Can you work these out from the model? Positions are in its coordinate system, mm. Round coordinates to 2 decimals unless told otherwise and drop trailing zeros. Loops run counter-clockwise (first coordinate to the right, second up) from the corner with the lowest first, then second, coordinate; pieces in that order, holes last. Notation, with made-up numbers: M 38,56 L 77,56 A16 cw 77,72 Z; hole C -14,87 d2. An arc over 180 degrees is marked long. Return JSON: item names as keys, results as strings.
```python
from build123d import *

# Parameters (mm, degrees)
SKETCH_1_W      = 42.566219829
SKETCH_1_H      = 4.687941776
SKETCH_1_W_2    = 6.910818326
SKETCH_1_H_2    = 4.318604229
SKETCH_1_W_3    = 5.015201163
SKETCH_1_H_3    = 4.736132542
SKETCH_1_W_4    = 61.28040068
SKETCH_1_H_4    = 1.827886604
EXTRUDE_1_DEPTH = 2
FILLET_1_R      = 2
FILLET_2_R      = 2


with BuildPart() as part:
    # 草图1 → 凸台-拉伸1 (new body)
    with BuildSketch(Plane(origin=(0, 0, 0), x_dir=(1, 0, 0), z_dir=(0, 1, 0))):
        Polygon((-50.243578821, 63.5), (-50.243578821, -53.4162), (-42.80979865, -53.4162), (-42.80979865, -49.097595771), (-42.80979865, -39.017252134), (-42.80979865, -34.329310358), (-42.80979865, 28.04266881), (-42.80979865, 32.778801352), (-42.80979865, 63.5), align=None)
        with Locations((-21.526688736, -36.673281246)):
            Rectangle(SKETCH_1_W, SKETCH_1_H)
        with Locations((-39.354389487, -51.256897886)):
            Rectangle(SKETCH_1_W_2, SKETCH_1_H_2)
        with Locations((-33.391379742, -51.256897886)):
            Rectangle(SKETCH_1_W_3, SKETCH_1_H_2)
        Polygon((-35.898980324, -53.4162), (-35.898980324, -63.5), (-30.883779161, -63.5), (-30.883779161, -62.190126209), (-30.883779161, -60.362239605), (-30.883779161, -53.4162), align=None)
        with Locations((21.039531094, -36.673281246)):
            Rectangle(SKETCH_1_W, SKETCH_1_H)
        Polygon((30.396621519, -62.190126209), (30.396621519, -63.5), (35.411822682, -63.5), (35.411822682, -53.4162), (30.396621519, -53.4162), (30.396621519, -60.362239605), align=None)
        with Locations((38.867231845, -51.256897886)):
            Rectangle(SKETCH_1_W_2, SKETCH_1_H_2)
        with Locations((32.904222101, -51.256897886)):
            Rectangle(SKETCH_1_W_3, SKETCH_1_H_2)
        Polygon((49.756421179, 63.5), (42.322641008, 63.5), (42.322641008, 32.778801352), (42.322641008, 28.04266881), (42.322641008, -34.329310358), (42.322641008, -39.017252134), (42.322641008, -49.097595771), (42.322641008, -53.4162), (49.756421179, -53.4162), align=None)
        with Locations((21.039531094, 30.410735081)):
            Rectangle(SKETCH_1_W, SKETCH_1_H_3)
        with Locations((-21.526688736, 30.410735081)):
            Rectangle(SKETCH_1_W, SKETCH_1_H_3)
        with Locations((-0.243578821, -61.276182907)):
            Rectangle(SKETCH_1_W_4, SKETCH_1_H_4)
    extrude(amount=EXTRUDE_1_DEPTH)

    # 圆角1
    fillet_1_edges = [part.edges().sort_by_distance(p)[0] for p in [
        (42.322641008, 1, -28.04266881),
        (-42.80979865, 1, -28.04266881),
        (-42.80979865, 1, 34.329310358),
        (42.322641008, 1, 34.329310358),
        (-42.80979865, 1, 39.017252134),
        (-42.80979865, 1, 49.097595771),
        (-30.883779161, 1, 49.097595771),
        (-30.883779161, 1, 60.362239605),
        (30.396621519, 1, 49.097595771),
        (42.322641008, 1, 49.097595771),
        (42.322641008, 1, 39.017252134),
        (-42.80979865, 1, -32.778801352),
        (42.322641008, 1, -32.778801352),
        (35.411822682, 1, 53.4162),
    ]]
    fillet(fillet_1_edges, radius=FILLET_1_R)

    # 圆角2
    fillet_2_edges = [part.edges().sort_by_distance(p)[0] for p in [
        (-35.898980324, 1, 63.5),
        (-35.898980324, 1, 53.4162),
        (-50.243578821, 1, 53.4162),
        (49.756421179, 1, 53.4162),
        (35.411822682, 1, 63.5),
    ]]
    fillet(fillet_2_edges, radius=FILLET_2_R)


solid = part.part
```
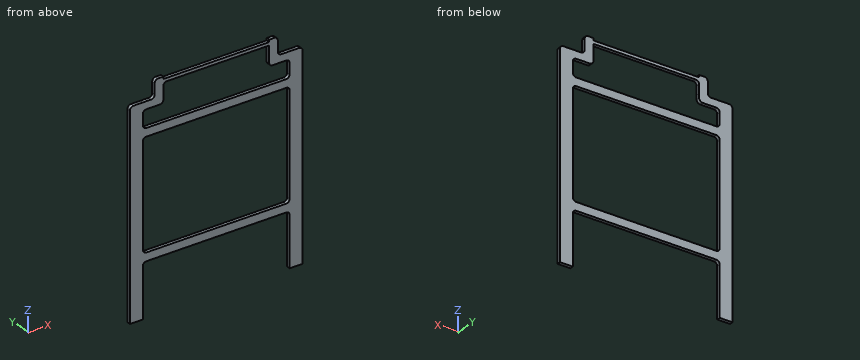
Q1. I'm going to push flat-ended pins straight in: pin 1 Ø1 at (y, z) = (1, 63) entering from -X; pin 2 Ø0.7 at (y, z) = (1, 63) entering from +X; pin 3 Ø1 at (x, z) = (21, 33) entering from +Y; pin 4 Ø0.6 at (x, y) = (-6.5, 0.5) entering from -Z. Where does each tip first touch, or does it pass through?
Results:
{"pin 1": "stops at x = -35.63", "pin 2": "stops at x = 35.05", "pin 3": "passes through", "pin 4": "stops at z = -32.78"}
Q2. Suppose I cut it at B-B, the plane x = 9. Please give me the cut outline in (y, z), plus the area to 3 significant figures.
Results:
{"outline": "M 0,-32.78 L 2,-32.78 L 2,-28.04 L 0,-28.04 Z; M 0,34.33 L 2,34.33 L 2,39.02 L 0,39.02 Z; M 0,60.36 L 2,60.36 L 2,62.19 L 0,62.19 Z", "area": "22.5 mm2"}
Q3. Suppose I cut it at A-A, the plane z = 14. Please give me the cut outline in (x, y).
Results:
{"outline": "M -50.24,0 L -42.81,0 L -42.81,2 L -50.24,2 Z; M 42.32,0 L 49.76,0 L 49.76,2 L 42.32,2 Z"}
Q4. If I drill on line 1 along Z through (x, y) = (29, 0.1); line 2 along Z through (x, y) = (-34, 0.8); line 3 along X through (y, z) = (1.4, -5), over which ranges is the centre line in solid material (lowest first)?
Results:
{"line 1": "z = -32.78 to -28.04, 34.33 to 39.02, 60.36 to 62.19", "line 2": "z = -32.78 to -28.04, 34.33 to 39.02, 49.1 to 63.5", "line 3": "x = -50.24 to -42.81, 42.32 to 49.76"}
Q5. Suppose I cut it at C-C, the plane y = 1.2. State how many separate pieces and enclosed holes the cut face has, plus the area to 3 significant figures.
Results:
{"separate pieces": "1", "enclosed holes": "2", "area": "2,860 mm2"}
